```python
from build123d import *

# Parameters (mm, degrees)
F0_R     = 20.6375
F0_R_2   = 20.0375
F1_DEPTH = 12.7
F2_R     = 21.2375
F3_DEPTH = 0.7


# Not quite as in the source:
# - a fillet or chamfer that OpenCascade refuses, or shapes differently, is made with other operations: its cross-section is extruded or revolved along the edge and cut away or added


with BuildPart() as f1:
    # F0 (on Top) → F1 (new body)
    with BuildSketch(Plane.XY):
        Circle(F0_R)
        Circle(F0_R_2, mode=Mode.SUBTRACT)
    extrude(amount=F1_DEPTH)

    # F2 (on Top) → F3 (join)
    with BuildSketch(Plane.XY):
        Circle(F2_R)
    extrude(amount=-F3_DEPTH)

    # F4: chamfer of 1 on 1 edges, made by hand

    # F4_s1 → F4_t2 (revolve, cut)
    with BuildSketch(Plane.XZ):
        Polygon((20.6375, 11.7), (19.6375, 12.7), (20.6375, 12.7), align=None)
    revolve(axis=Axis((0, 0, 12.7), (0, 0, 1)), mode=Mode.SUBTRACT)


solid = f1.part
```
The model under review builds one solid part; all positions refer to its coordinate system, in mm. A direction names the side the tool comes from. Round coordinates to 2 decimals unless told otherwise and drop trailing zeros. Order: outer loops, then holes, each group sorted by start corner. A loop starts at its lowest first (then second) coordinate and runs counter-clockwise, first axis right, second up. Notation, with made-up numbers: M 13.25,-7 L 24.25,-7 A15 cw 24.25,22 Z; hole C 58.25,-30.75 d1. An arc over 180 degrees is marked long. Use a Markdown table: item, result.
1) Tool access review of faces 1 (the face through (0, 0, 0)), 2 (the face through (0, 0, -0.7)): name each direction out of +Z, -Z, +X, -X, +Y, -Y from which nothing blocks a thin tool from reaching the whole face with its end or side.
Report:
| item | result |
|---|---|
| face 1 | +Z |
| face 2 | -Z, +X, -X, +Y, -Y |
2) Wall thickness on line 1 along Y through (x, z) = (0, 9); line 2 along Z through (x, y) = (4, 7.5); line 3 along Y through (x, z) = (15, 3.5): over which ranges is each line inside the solid? List them lowest first. Write a range as [from, to].
Report:
| item | result |
|---|---|
| line 1 | [-20.64, -20.04], [20.04, 20.64] |
| line 2 | [-0.7, 0] |
| line 3 | [-14.17, -13.29], [13.29, 14.17] |
3) Insertion check: pin 1 (2 mm diameter, centred on y = 13.5, z = 8.5, fed in from -X); pin 2 (3 mm diameter, centred on y = -4, z = 7, fed in from -X); pin 3 (4 mm diameter, centred on x = -14, y = -6, fed in from +Z). Each pin has a flat end and moves straight along its axis. Give the tip position at first contact, or say it passes through.
Report:
| item | result |
|---|---|
| pin 1 | x = -16.42 |
| pin 2 | x = -20.49 |
| pin 3 | z = 0 |
4) Consider section C-C (z = 4). Write out the cut boundary in (x, y) (1 decimal).
Report:
| item | result |
|---|---|
| outline | C 0,0 d41.3; hole C 0,0 d40.1 |
5) Consider section A-A (x = 0). Write out the cut boundary in (y, z), then the cut area to 3 significant figures.
Report:
| item | result |
|---|---|
| outline | M -21.24,-0.7 L 21.24,-0.7 L 21.24,0 L 20.64,0 L 20.64,11.7 L 20.04,12.3 L 20.04,0 L -20.04,0 L -20.04,12.3 L -20.64,11.7 L -20.64,0 L -21.24,0 Z |
| area | 44.1 mm^2 |
6) Draft analysis for pull direction X (two halves, no side actions). For faces 3 (the face through (-2.608, 19.867, 6.064)), 4 (the face through (-4.474, -20.147, 5.768)), 5 (the face through (-3.2, 20.6, 0)), state which applies: released by +X, released by -X, zero draft, split by the parting line, or undercut.
Report:
| item | result |
|---|---|
| face 3 | undercut |
| face 4 | split by the parting line |
| face 5 | zero draft |
